Work out the finished part from the listing and answer in its coordinate system (mm). A direction names the side the tool comes from. Round coordinates to 2 decimals unless told otherwise and drop trailing zeros. Order: outer loops, then holes, each group sorted by start corner. A loop starts at its lowest first (then second) coordinate and runs counter-clockwise, first axis right, second up. Notation, with made-up numbers: (4, 77) - (48, 77) arc R14 cw to (48, 96) - close; hole circle Ø9 at (19, 59). An arc over 180 degrees is marked (long way). Use CSV: the item, a comma, the result in double quotes.
from build123d import *

# Parameters (mm, degrees)
SKETCH005_R     = 14.5
SKETCH005_R_2   = 1.7
PAD004_DEPTH    = 2.6
SKETCH006_R     = 3.6
POCKET001_DEPTH = 1.4
FILLET_R        = 2
SKETCH010_R     = 5.25
SKETCH010_R_2   = 1.7
PAD007_DEPTH    = 0.6


with BuildPart() as part:
    # Sketch005 → Pad004 (new body)
    with BuildSketch(Plane.XY):
        Circle(SKETCH005_R)
        Circle(SKETCH005_R_2, mode=Mode.SUBTRACT)
    extrude(amount=PAD004_DEPTH)

    # Sketch006 (on Face4 of Pad004) → Pocket001 (cut)
    with BuildSketch(Plane.XY.offset(2.6)):
        Circle(SKETCH006_R)
    extrude(amount=-POCKET001_DEPTH, mode=Mode.SUBTRACT)

    # Fillet
    fillet_edges = [part.edges().sort_by_distance(p)[0] for p in [
        (-14.5, 0, 2.6),
    ]]
    fillet(fillet_edges, radius=FILLET_R)

    # Sketch010 (on Face3 of Fillet) → Pad007 (join)
    with BuildSketch(Plane(origin=(0, 0, 0), x_dir=(1, 0, 0), z_dir=(0, 0, -1))):
        Circle(SKETCH010_R)
        Circle(SKETCH010_R_2, mode=Mode.SUBTRACT)
    extrude(amount=PAD007_DEPTH)


solid = part.part
(1) The mould has two halves that part along Y. Classify faces 4 (the cylindrical face through (-0.37, 1.66, 0.31)), 5 (the flat face through (3, -3, 2.6)), 6 (the flat face through (1, -2, 1.2)), 7 (the cylindrical face through (6.691, -12.864, 0.296)): released by +Y, released by -Y, zero draft, split by the parting line, or undercut.
Findings below:
face 4,"undercut"
face 5,"zero draft"
face 6,"undercut"
face 7,"split by the parting line"
(2) Find section A-A (y = 0). Determine the outline of the cut face in (x, z), and give its area (3 significant figures).
Findings below:
outline,"(-14.5, 0) - (-5.25, 0) - (-5.25, -0.6) - (-1.7, -0.6) - (-1.7, 1.2) - (-3.6, 1.2) - (-3.6, 2.6) - (-12.5, 2.6) arc R2 ccw to (-14.5, 0.6) - close; (1.7, -0.6) - (5.25, -0.6) - (5.25, 0) - (14.5, 0) - (14.5, 0.6) arc R2 ccw to (12.5, 2.6) - (3.6, 2.6) - (3.6, 1.2) - (1.7, 1.2) - close"
area,"63.8 mm²"
(3) Each of these flat-tipped pins is pushed along its axis until it touches: pin 1 (1.5 mm diameter, centred on y = 1.5, z = 0, fed in from +X); pin 2 (3.5 mm diameter, centred on x = 0, y = 0, fed in from +Z); pin 3 (1.5 mm diameter, centred on x = -6, z = 2, fed in from -Y). Where does it stop, or does it pass through?
Findings below:
pin 1,"stops at x = 14.48"
pin 2,"stops at z = 1.2"
pin 3,"stops at y = -13.22"
(4) Find the intervals of material crossed by L1, parallel to Y at x = 0, z = 0.4; L2, parallel to Y at x = 0, z = 2.1; L3, parallel to X at y = 0.75, z = 1.8, in increasing order. Write a range as from..to.
Findings below:
L1,"y = -14.5..-1.7, 1.7..14.5"
L2,"y = -13.82..-3.6, 3.6..13.82"
L3,"x = -14.08..-3.52, 3.52..14.08"
(5) For faces 1 (the flat face through (2, 0, -0.6)), 2 (the flat face through (6, 0, 0)), 3 (the cylindrical face through (3.434, 1.081, 1.91)), determine the directions among +Z, -Z, +X, -X, +Y, -Y from which every point of the face is accessible in a straight line to the end or side of a thin tool.
Findings below:
face 1,"-Z, +X, -X, +Y, -Y"
face 2,"-Z"
face 3,"+Z"
